Geometry: final body of the model. Coordinates: model frame, mm. Give positions to 0.01 mm unless a question says otherwise; leave off trailing zeros. Write each loop counter-clockwise with the first axis right and the second up, starting at its lowest first coordinate (ties: lowest second). Pieces come first, ordered by that corner, then holes. Notation, with made-up numbers: M 4.25,-37 L 32.25,-37 A23 cw 32.25,-22 Z; hole C -39,1 d10. An arc over 180 degrees is marked long. Use one line per item in the form item = value. Start each with the question number.
Item 1: Material intervals for line 1 along X through (y, z) = (143, 4.4); line 2 along X through (y, z) = (119, 3.45); line 3 along Y through (x, z) = (-12.5, 0.55), sorted ascending. Write a range as from..to.
Item 2: Section query A-A on z = 1.7. Give the number of separate pieces and of enclosed holes in the cut face, then the cut area to 3 significant figures.
Item 3: Section query C-C on x = -27. Return loops of the section in (y, z).
Item 4: Section query B-B on y = 50. Return loops of the section in (x, z), then the cut area to 3 significant figures.
Item 5: Contact query for flat-ended pins moving along their axis: P1, Ø2, axis at y = 136, z = 3, coming from the +X side; P2, Ø2.5, axis at x = -32, z = 3.5, coming from the -Y side; P3, Ø2.5, axis at y = -3, z = 2.5, coming from the +X side. Output: stop coordinate, or through.
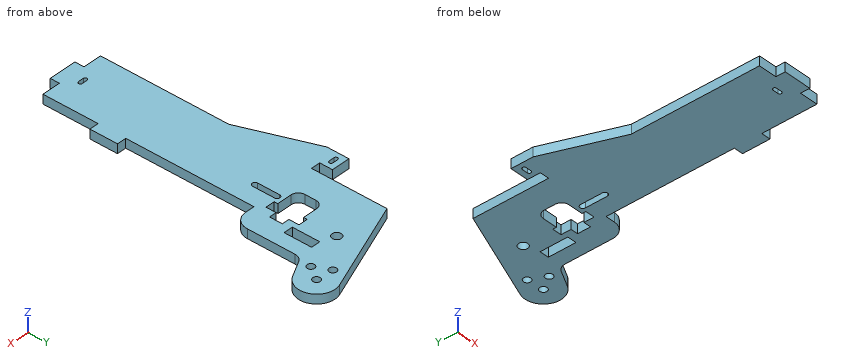
from build123d import *

# Parameters (mm, degrees)
SKETCH2_R           = 2
BOSS_EXTRUDE1_DEPTH = 5
SKETCH3_R           = 2.5
CUT_EXTRUDE1_DEPTH  = 181.287193762
BOSS_EXTRUDE2_DEPTH = 5
FILLET1_R           = 5
CUT_EXTRUDE2_DEPTH  = 184.789205979
SKETCH6_W           = 5
SKETCH6_H           = 15
CUT_EXTRUDE3_DEPTH  = 184.789205979
FILLET2_R           = 4


with BuildPart() as part:
    # Sketch2 → Boss-Extrude1 (new body)
    with BuildSketch(Plane.XY):
        with BuildLine():
            Line((16.34105486, 176.093079286), (-35, 155.907958626))
            Line((-35, 155.907958626), (-35, 0))
            Line((-35, 0), (-25, 0))
            Line((-25, 0), (-25, -5))
            Line((-25, -5), (-10, -5))
            Line((-10, -5), (-10, 0))
            Line((-10, 0), (0, 0))
            Line((0, 0), (0, 30))
            Line((0, 30), (5, 30))
            Line((5, 30), (5, 45))
            Line((5, 45), (0, 45))
            Line((0, 45), (0, 114.786515986))
            Line((0, 114.786515986), (5, 114.786515986))
            ThreePointArc((5, 114.786515986), (10.656854249, 117.129661736), (13, 122.786515986))
            Line((13, 122.786515986), (13, 151.786515986))
            Line((13, 151.786515986), (24.666554357, 157.942123953))
            ThreePointArc((24.666554357, 157.942123953), (29.089450696, 170.955674898), (16.34105486, 176.093079286))
        make_face()
        with Locations((20, 166.786515986)):
            Circle(SKETCH2_R, mode=Mode.SUBTRACT)
        with Locations((10.78085199, 167.370162539)):
            Circle(SKETCH2_R, mode=Mode.SUBTRACT)
        with Locations((14.884973253, 159.094322884)):
            Circle(SKETCH2_R, mode=Mode.SUBTRACT)
    extrude(amount=BOSS_EXTRUDE1_DEPTH)

    # Sketch3 → Cut-Extrude1 (cut, through all)
    with BuildSketch(Plane.XY.offset(5)):
        with Locations((-7.5, 153.1488261)):
            Circle(SKETCH3_R)
        Polygon((-3, 136.647544915), (-3, 131.147544915), (1, 131.147544915), (1, 124.147544915), (-3, 124.147544915), (-3, 118.647544915), (-8, 118.647544915), (-8, 120.647544915), (-20, 120.647544915), (-20, 134.647544915), (-8, 134.647544915), (-8, 136.647544915), align=None)
    extrude(amount=-CUT_EXTRUDE1_DEPTH, mode=Mode.SUBTRACT)

    # Sketch4 → Boss-Extrude2 (add)
    with BuildSketch(Plane(origin=(0, 0, 0), x_dir=(-1, 0, 0), z_dir=(0, 0, -1))):
        Polygon((40, 114.786515986), (35, 114.786515986), (35, 69.786515986), (50, 109.786515986), (50, 121.786515986), (40, 121.786515986), align=None)
    extrude(amount=-BOSS_EXTRUDE2_DEPTH)

    # Fillet1
    fillet1_edges = [part.edges().sort_by_distance(p)[0] for p in [
        (13, 151.786515986, 2.5),
    ]]
    fillet(fillet1_edges, radius=FILLET1_R)

    # Sketch5 → Cut-Extrude2 (cut, through all)
    with BuildSketch(Plane.XY.offset(5)):
        with BuildLine():
            Line((-10, 117.147544915), (-10, 105.147544915))
            ThreePointArc((-10, 105.147544915), (-11.5, 103.647544915), (-13, 105.147544915))
            Line((-13, 105.147544915), (-13, 117.147544915))
            ThreePointArc((-13, 117.147544915), (-11.5, 118.647544915), (-10, 117.147544915))
        make_face()
        with BuildLine():
            Line((-43.5, 116.786515986), (-46.5, 116.786515986))
            ThreePointArc((-46.5, 116.786515986), (-47.5, 117.786515986), (-46.5, 118.786515986))
            Line((-46.5, 118.786515986), (-43.5, 118.786515986))
            ThreePointArc((-43.5, 118.786515986), (-42.5, 117.786515986), (-43.5, 116.786515986))
        make_face()
        with BuildLine():
            Line((-19, 7), (-16, 7))
            ThreePointArc((-16, 7), (-15, 6), (-16, 5))
            Line((-16, 5), (-19, 5))
            ThreePointArc((-19, 5), (-20, 6), (-19, 7))
        make_face()
    extrude(amount=-CUT_EXTRUDE2_DEPTH, mode=Mode.SUBTRACT)

    # Sketch6 → Cut-Extrude3 (cut, through all)
    with BuildSketch(Plane(origin=(0, 0, 0), x_dir=(-1, 0, 0), z_dir=(0, 0, -1))):
        with Locations((-2.5, 143.148799484)):
            Rectangle(SKETCH6_W, SKETCH6_H)
    extrude(amount=-CUT_EXTRUDE3_DEPTH, mode=Mode.SUBTRACT)

    # Fillet2
    fillet2_edges = [part.edges().sort_by_distance(p)[0] for p in [
        (-20, 134.647544915, 2.5),
        (-20, 120.647544915, 2.5),
    ]]
    fillet(fillet2_edges, radius=FILLET2_R)


solid = part.part
Answer sheet:
q1.line_1 = -35..0, 5..13
q1.line_2 = -50..-40, -35..-8, -3..12.05
q1.line_3 = -5..104.03, 118.27..120.65, 134.65..164.75
q2.separate_pieces = 1
q2.enclosed_holes = 9
q2.area = 6,870 mm2
q3.outline = M 0,0 L 159.05,0 L 159.05,5 L 0,5 Z
q4.outline = M -35,0 L 0,0 L 0,5 L -35,5 Z
q4.area = 175 mm2
q5.P1 = 13
q5.P2 = 0
q5.P3 = -10
